from build123d import *

# Parameters (mm, degrees)
SKETCH1_W           = 20
SKETCH1_H           = 42
BOSS_EXTRUDE1_DEPTH = 69.85
FILLET1_R           = 6.35
SKETCH3_W           = 42
SKETCH3_H           = 42
BOSS_EXTRUDE2_DEPTH = 6.35
SKETCH4_W           = 16
SKETCH4_H           = 24
CUT_EXTRUDE2_DEPTH  = 80.252902155
SKETCH8_R           = 4
CUT_EXTRUDE5_DEPTH  = 80.252902155
FILLET2_R           = 6
FILLET3_R           = 4
FILLET4_R           = 3
SKETCH9_W           = 11
SKETCH9_H           = 42
CUT_EXTRUDE6_DEPTH  = 85.166635314
SKETCH10_R          = 4.000000001
BOSS_EXTRUDE3_DEPTH = 1
SKETCH11_R          = 2.5
BOSS_EXTRUDE4_DEPTH = 6
SKETCH12_W          = 20
SKETCH12_H          = 27.5
BOSS_EXTRUDE5_DEPTH = 6.35
SKETCH13_W          = 20
SKETCH13_H          = 4
BOSS_EXTRUDE6_DEPTH = 5.08
SKETCH2_R           = 7.5
CUT_EXTRUDE1_DEPTH  = 76.227580713
FILLET5_R           = 3


with BuildPart() as part:
    # Sketch1 → Boss-Extrude1 (new body)
    with BuildSketch(Plane(origin=(0, 0, 0), x_dir=(1, 0, 0), z_dir=(0, 1, 0))):
        Rectangle(SKETCH1_W, SKETCH1_H)
    extrude(amount=BOSS_EXTRUDE1_DEPTH)

    # Fillet1
    fillet1_edges = [part.edges().sort_by_distance(p)[0] for p in [
        (10, 34.925, 21),
        (-10, 34.925, 21),
    ]]
    fillet(fillet1_edges, radius=FILLET1_R)

    # Sketch3 → Boss-Extrude2 (add)
    with BuildSketch(Plane(origin=(0, 0, -21), x_dir=(-1, 0, 0), z_dir=(0, 0, -1))):
        with Locations((0, 34.925)):
            Rectangle(SKETCH3_W, SKETCH3_H)
    extrude(amount=-BOSS_EXTRUDE2_DEPTH)

    # Sketch4 → Cut-Extrude2 (cut, through all)
    with BuildSketch(Plane(origin=(10, 0, 0), x_dir=(0, 0, -1), z_dir=(1, 0, 0))):
        with Locations((6.65, 34.925)):
            Rectangle(SKETCH4_W, SKETCH4_H)
    extrude(amount=-CUT_EXTRUDE2_DEPTH, mode=Mode.SUBTRACT)

    # Sketch8 → Cut-Extrude5 (cut, through all)
    with BuildSketch(Plane(origin=(10, 0, 0), x_dir=(0, 0, -1), z_dir=(1, 0, 0))):
        with Locations((7.318215362, 60.425)):
            Circle(SKETCH8_R)
        with Locations((7.318215362, 9.425)):
            Circle(SKETCH8_R)
    extrude(amount=-CUT_EXTRUDE5_DEPTH, mode=Mode.SUBTRACT)

    # Fillet2
    fillet2_edges = [part.edges().sort_by_distance(p)[0] for p in [
        (0, 0, -21),
        (0, 69.85, -21),
    ]]
    fillet(fillet2_edges, radius=FILLET2_R)

    # Fillet3
    fillet3_edges = [part.edges().sort_by_distance(p)[0] for p in [
        (-21, 13.925, -17.825),
        (21, 55.925, -17.825),
        (-21, 55.925, -17.825),
        (21, 13.925, -17.825),
    ]]
    fillet(fillet3_edges, radius=FILLET3_R)

    # Fillet4
    fillet4_edges = [part.edges().sort_by_distance(p)[0] for p in [
        (0, 22.925, 1.35),
        (0, 46.925, -14.65),
        (0, 22.925, -14.65),
        (0, 46.925, 1.35),
    ]]
    fillet(fillet4_edges, radius=FILLET4_R)

    # Sketch9 → Cut-Extrude6 (cut, through all)
    with BuildSketch(Plane(origin=(0, 0, -21), x_dir=(-1, 0, 0), z_dir=(0, 0, -1))):
        with Locations((-15.5, 34.925)):
            Rectangle(SKETCH9_W, SKETCH9_H)
        with Locations((15.5, 34.925)):
            Rectangle(SKETCH9_W, SKETCH9_H)
    extrude(amount=-CUT_EXTRUDE6_DEPTH, mode=Mode.SUBTRACT)

    # Sketch10 → Boss-Extrude3 (add)
    with BuildSketch(Plane.XY.offset(-14.65)):
        with Locations((0, 34.925)):
            Circle(SKETCH10_R)
    extrude(amount=BOSS_EXTRUDE3_DEPTH)

    # Sketch11 → Boss-Extrude4 (add)
    with BuildSketch(Plane.XY.offset(-13.65)):
        with Locations((0, 34.925)):
            Circle(SKETCH11_R)
    extrude(amount=BOSS_EXTRUDE4_DEPTH)

    # Sketch12 → Boss-Extrude5 (add)
    with BuildSketch(Plane.XY.offset(21)):
        with Locations((0, 34.925)):
            Rectangle(SKETCH12_W, SKETCH12_H)
    extrude(amount=-BOSS_EXTRUDE5_DEPTH)

    # Sketch13 → Boss-Extrude6 (add)
    with BuildSketch(Plane.XY.offset(21)):
        with Locations((0, 46.675)):
            Rectangle(SKETCH13_W, SKETCH13_H)
        with Locations((0, 23.175)):
            Rectangle(SKETCH13_W, SKETCH13_H)
    extrude(amount=BOSS_EXTRUDE6_DEPTH)

    # Sketch2 → Cut-Extrude1 (cut, through all)
    with BuildSketch(Plane(origin=(0, 69.85, 0), x_dir=(1, 0, 0), z_dir=(0, 1, 0))):
        with Locations(Location((0, -11.254449914, 0), (0, 0, 270))):
            Circle(SKETCH2_R)
    extrude(amount=-CUT_EXTRUDE1_DEPTH, mode=Mode.SUBTRACT)

    # Fillet5
    fillet5_edges = [part.edges().sort_by_distance(p)[0] for p in [
        (0, 21.175, 26.08),
        (0, 48.675, 26.08),
    ]]
    fillet(fillet5_edges, radius=FILLET5_R)


solid = part.part
Design review of the part built by this model. Coordinates are the model's own, in mm. A direction names the side the tool comes from. Give positions to 0.01 mm unless a question says otherwise; leave off trailing zeros. Write each loop counter-clockwise with the first axis right and the second up, starting at its lowest first coordinate (ties: lowest second). Pieces come first, ordered by that corner, then holes. Notation, with made-up numbers: M 79,42.5 L 125,42.5 A22 ccw 125,56.5 Z; hole C -28,-5 d6. An arc over 180 degrees is marked long. Return JSON: item names as keys, results as strings. Group by question number.
Item 1: Take a section at C-C (y = 7). Give the boundary of the cut face in (x, z).
Item 2: Clearance check with flat-ended pins moving along their axes: pin 1 Ø1.5 at (x, y) = (6, 33.5) entering from +Z; pin 2 Ø4 at (x, z) = (-2.5, 24) entering from -Y (3 decimals). State where each tip first meets the part, or that it passes through.
Item 3: Take a section at A-A (y = 53.5). Give the boundary of the cut face in (x, z), plus the area to 3 significant figures.
Item 4: Tool access review of faces 1 (the flat face through (0, 22.925, -7)), 2 (the flat face through (0, 35, 21)), 3 (the flat face through (0, 59, 21)): name each direction out of +Z, -Z, +X, -X, +Y, -Y from which nothing blocks a thin tool from reaching the whole face with its end or side.
Item 5: Take a section at D-D (z = -5). Give the boundary of the cut face in (x, y) (3 decimals).
Item 6: The part is to be moulded in two halves that separate along Y. For faces 4 (the flat face through (-0.8, 21.175, 21.4)), 5 (the flat face through (0, 11, 21)), 6 (the flat face through (0, 35, -7.65)), say which applies: pulls with the +Y half, pulls with the -Y half, needs draft (parallel to the pull), parting line crosses it, or undercut.
Item 7: Wall thickness on line 1 along Y through (x, z) = (3.5, -7.5) (3 decimals); line 2 along Z through (x, y) = (-1.25, 34.5); line 3 along Z through (x, y) = (0.5, 50): over which ranges is each line inside the solid? List them lowest first.
Item 8: Take a section at B-B (z = -12.5). Give the boundary of the cut face in (x, y) (3 decimals), plus the area to 3 significant figures.
Return value:
{
 "1": {"outline": "M -10,-21 L 10,-21 L 10,-10.5 L -10,-10.5 Z; M -10,-4.14 L 10,-4.14 L 10,14.65 A6.35 ccw 3.65,21 L -3.65,21 A6.35 ccw -10,14.65 Z; hole C 0,11.25 d15"},
 "2": {"pin 1": "stops at z = 21", "pin 2": "stops at y = 21.175"},
 "3": {"outline": "M -10,-21 L 10,-21 L 10,14.65 A6.35 ccw 3.65,21 L -3.65,21 A6.35 ccw -10,14.65 Z; hole C 0,11.25 d15", "area": "646 mm2"},
 "4": {"face 1": "+X, -X", "face 2": "+Z, +X, -X", "face 3": "+Z, +X, -X, +Y"},
 "5": {"outline": "M -10,0 L 10,0 L 10,6.165 L -10,6.165 Z; M -10,12.685 L 10,12.685 L 10,22.925 L -10,22.925 Z; M -10,46.925 L 10,46.925 L 10,57.165 L -10,57.165 Z; M -10,63.685 L 10,63.685 L 10,69.85 L -10,69.85 Z"},
 "6": {"face 4": "pulls with the -Y half", "face 5": "needs draft", "face 6": "undercut"},
 "7": {"line 1": "y = 0 to 5.429, 13.421 to 22.925, 46.925 to 56.429, 64.421 to 69.85", "line 2": "z = -21 to -7.65, 1.35 to 3.86, 18.65 to 21", "line 3": "z = -21 to 3.77, 18.74 to 21"},
 "8": {"outline": "M -10,0 L 10,0 L 10,23.048 L -10,23.048 Z; M -10,46.802 L 10,46.802 L 10,69.85 L -10,69.85 Z; C 0,34.925 d5", "area": "942 mm2"}
}
